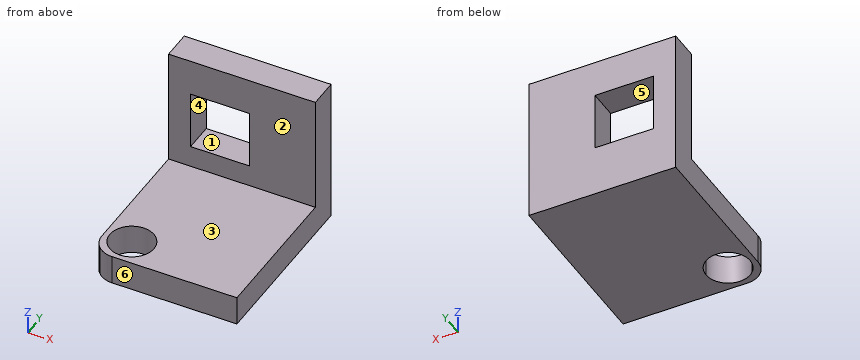
from build123d import *

# Parameters (mm, degrees)
F1_DEPTH = 20
F2_W     = 100
F2_H     = 100
F2_W_2   = 40
F2_H_2   = 40
F3_DEPTH = 20


with BuildPart() as f1:
    # F0 (on Top) → F1 (new body)
    with BuildSketch(Plane.XY):
        with BuildLine():
            Line((100, 0), (0, 0))
            Line((0, 0), (0, -85))
            ThreePointArc((0, -85), (1.141807, -90.740251), (4.393398, -95.606602))
            ThreePointArc((4.393398, -95.606602), (9.259749, -98.858193), (15, -100))
            Line((15, -100), (100, -100))
            Line((100, -100), (100, 0))
        make_face()
        with BuildLine():
            ThreePointArc((33.508259, -81.381075), (24.284639, -95.224247), (7.957134, -92.042866))
            ThreePointArc((7.957134, -92.042866), (12.731878, -67.537902), (33.508259, -81.381075))
        make_face(mode=Mode.SUBTRACT)
    extrude(amount=F1_DEPTH)

    # F2 (on Front) → F3 (join)
    with BuildSketch(Plane.XZ):
        with Locations((50, 50)):
            Rectangle(F2_W, F2_H)
        with Locations((35, 55)):
            Rectangle(F2_W_2, F2_H_2, mode=Mode.SUBTRACT)
    extrude(amount=-F3_DEPTH)


solid = f1.part
Verification items for the finished model (mm, model axes). Face numbers are marked on the shaded views. A direction names the side the tool comes from. Coordinates: 2 decimals unless noted, no trailing zeros. Loops run counter-clockwise (first coordinate to the right, second up) from the corner with the lowest first, then second, coordinate; pieces in that order, holes last. Notation, with made-up numbers: (83, -14.75) -> (136, -14.75) arc R17 cw to (136, 5.25) -> close; hole circle Ø6 at (86, 70.25). An arc over 180 degrees is marked (long way). Write each question's results on one line, items separated by ' | '.
Item 1: Section check C-C, the plane y = 13.5. Enter the section's corners in (x, z).
Found:
outline: (0, 0) -> (100, 0) -> (100, 100) -> (0, 100) -> close; hole (15, 35) -> (55, 35) -> (55, 75) -> (15, 75) -> close
Item 2: Section check A-A, the plane x = 46. Enter the section's corners in (y, z), plus the area to 3 significant figures.
Found:
outline: (-100, 0) -> (20, 0) -> (20, 35) -> (0, 35) -> (0, 20) -> (-100, 20) -> close; (0, 75) -> (20, 75) -> (20, 100) -> (0, 100) -> close | area: 3,200 mm2
Item 3: Mould release check, pull along Z, two halves, no side actions. Record for the marked faces 1, 2, 3 and 4: +Z half, -Z half, draft (parallel to the pull), parting line (faces both ways), or undercut.
Found:
face 1: undercut | face 2: draft | face 3: +Z half | face 4: undercut
Item 4: Gauge pin test, flat ends, axial feed: pin 1 (12 mm diameter, centred on x = 51.5, y = -27, fed in from -Z); pin 2 (8 mm diameter, centred on y = -87.5, z = 23.5, fed in from -X); pin 3 (10 mm diameter, centred on x = 60, y = -61, fed in from +Z). Record the tip position at first contact, or that the pin passes through.
Found:
pin 1: stops at z = 0 | pin 2: stops at x = 0.01 | pin 3: stops at z = 20
Item 5: Section check B-B, the plane z = 39. Enter the section's corners in (x, y).
Found:
outline: (0, 0) -> (15, 0) -> (15, 20) -> (0, 20) -> close; (55, 0) -> (100, 0) -> (100, 20) -> (55, 20) -> close
Item 6: Tool access check on the marked faces 5 and 6. Record the directions out of +Z, -Z, +X, -X, +Y, -Y that give a thin tool (end or side, any length) a straight path to the whole face; none if there is none.
Found:
face 5: +Y, -Y | face 6: +Z, -Z, +X, -X, -Y
Item 7: Material ranges on L1, parallel to Y at x = 5.5, z = 53, recorded low to high.
Found:
L1: y = 0 to 20
Item 8: Section check D-D, the plane x = 19. Enter the section's corners in (y, z).
Found:
outline: (-100, 0) -> (-96.37, 0) -> (-96.37, 20) -> (-100, 20) -> close; (-66.39, 0) -> (20, 0) -> (20, 35) -> (0, 35) -> (0, 20) -> (-66.39, 20) -> close; (0, 75) -> (20, 75) -> (20, 100) -> (0, 100) -> close
